from build123d import *

# Parameters (mm, degrees)
SKETCH1_W           = 130
SKETCH1_H           = 230
BOSS_EXTRUDE1_DEPTH = 2
EXTRUDE_THIN1_DEPTH = 0.5
SKETCH3_R           = 1.5
CUT_EXTRUDE1_DEPTH  = 133.113587492


with BuildPart() as part:
    # Sketch1 → Boss-Extrude1 (new body)
    with BuildSketch(Plane.XY):
        Rectangle(SKETCH1_W, SKETCH1_H)
    extrude(amount=BOSS_EXTRUDE1_DEPTH)

    # Sketch2 → Extrude-Thin1 (add)
    with BuildSketch(Plane.XY.offset(2)):
        with BuildLine():
            Line((58.95, 84.95), (63, 84.95))
            Line((63, 84.95), (63, -104.9))
            Line((63, -104.9), (58.95, -104.9))
            ThreePointArc((58.95, -104.9), (56.086217536, -106.086217536), (54.9, -108.95))
            Line((54.9, -108.95), (54.9, -113))
            Line((54.9, -113), (-54.9, -113))
            Line((-54.9, -113), (-54.9, -108.95))
            ThreePointArc((-54.9, -108.95), (-56.086217536, -106.086217536), (-58.95, -104.9))
            Line((-58.95, -104.9), (-63, -104.9))
            Line((-63, -104.9), (-63, 104.9))
            Line((-63, 104.9), (-58.95, 104.9))
            ThreePointArc((-58.95, 104.9), (-56.086217536, 106.086217536), (-54.9, 108.95))
            Line((-54.9, 108.95), (-54.9, 113))
            Line((-54.9, 113), (63, 113))
            Line((63, 113), (63, 93.05))
            Line((63, 93.05), (58.95, 93.05))
            ThreePointArc((58.95, 93.05), (54.9, 89), (58.95, 84.95))
        make_face()
        with BuildLine():
            Line((58.95, 83.95), (62, 83.95))
            Line((62, 83.95), (62, -103.9))
            Line((62, -103.9), (58.95, -103.9))
            ThreePointArc((58.95, -103.9), (55.379110755, -105.379110755), (53.9, -108.95))
            Line((53.9, -108.95), (53.9, -112))
            Line((53.9, -112), (-53.9, -112))
            Line((-53.9, -112), (-53.9, -108.95))
            ThreePointArc((-53.9, -108.95), (-55.379110755, -105.379110755), (-58.95, -103.9))
            Line((-58.95, -103.9), (-62, -103.9))
            Line((-62, -103.9), (-62, 103.9))
            Line((-62, 103.9), (-58.95, 103.9))
            ThreePointArc((-58.95, 103.9), (-55.379110755, 105.379110755), (-53.9, 108.95))
            Line((-53.9, 108.95), (-53.9, 112))
            Line((-53.9, 112), (62, 112))
            Line((62, 112), (62, 94.05))
            Line((62, 94.05), (58.95, 94.05))
            ThreePointArc((58.95, 94.05), (53.9, 89), (58.95, 83.95))
        make_face(mode=Mode.SUBTRACT)
    extrude(amount=EXTRUDE_THIN1_DEPTH)

    # Sketch3 → Cut-Extrude1 (cut, through all)
    with BuildSketch(Plane.XY.offset(2)):
        with Locations((59, -109)):
            Circle(SKETCH3_R)
        with Locations((-59, -109)):
            Circle(SKETCH3_R)
        with Locations((-59, 109)):
            Circle(SKETCH3_R)
        with Locations((59, 89)):
            Circle(SKETCH3_R)
    extrude(amount=-CUT_EXTRUDE1_DEPTH, mode=Mode.SUBTRACT)


solid = part.part
Can you work these out from the model? Positions are in its coordinate system, mm. A direction names the side the tool comes from. Round coordinates to 2 decimals unless told otherwise and drop trailing zeros. Write each loop counter-clockwise with the first axis right and the second up, starting at its lowest first coordinate (ties: lowest second). Pieces come first, ordered by that corner, then holes. Notation, with made-up numbers: (26.5, 83.5) -> (82.5, 83.5) arc R22 cw to (82.5, 94.5) -> close; hole circle Ø1 at (76, 11.5). An arc over 180 degrees is marked (long way). One line per question, with ' | ' between items. Start each with the question number.
1) I need wall thicknesses on line 1 (Y direction, x = -59, z = 1.45); line 2 (X direction, y = -109, z = 0.55); line 3 (Y direction, x = 59, z = 1.2). Which ranges of each line are inside material? Lowest first, please. Write a range as [from, to].
2) Suppose I cut it at A-A on y = 100. Write out the boundary of the cut face in (x, z).
3) I'm going to push flat-ended pins straight in: P1, Ø0.6, axis at y = -110, z = 2.5, coming from the -X side; P2, Ø0.6, axis at y = 35.5, z = 2.5, coming from the +X side. Where does each tip first touch, or does it pass through?
4) On a 3-axis mill with a long thin cutter (end or side, diameter ignored), from which of +Z, -Z, +X, -X, +Y, -Y can I reach the whole of each face in a straight line? I mean faces 1 (the cylindrical face through (-56.055, -106.118, 2.246)), 2 (the cylindrical face through (-55.42, 105.34, 2.25)), 3 (the cylindrical face through (54.9, 89.1, 2.2)), 4 (the cylindrical face through (-56.118, 106.055, 2.246)). Say none if no direction works.
5) Suppose I cut it at B-B on x = 10.5. Write out the boundary of the cut face in (y, z), then the cut area to 3 significant figures.
6) If we mould it in two halves opening along X, with no side actions, what happens to faces 5 (the cylindrical face through (55.42, -105.34, 2.25)), 6 (the cylindrical face through (-55.34, -105.42, 2.25)), 7 (the cylindrical face through (56.118, -106.055, 2.246)), 8 (the flat face through (-1, 2, 0))? For each: released by +X, released by -X, zero draft, split by the parting line, or undercut.
Return value:
1) line 1: y = [-115, -110.5], [-107.5, 107.5], [110.5, 115] | line 2: x = [-65, -60.5], [-57.5, 57.5], [60.5, 65] | line 3: y = [-115, -110.5], [-107.5, 87.5], [90.5, 115]
2) outline: (-65, 0) -> (65, 0) -> (65, 2) -> (63, 2) -> (63, 2.5) -> (62, 2.5) -> (62, 2) -> (-62, 2) -> (-62, 2.5) -> (-63, 2.5) -> (-63, 2) -> (-65, 2) -> close
3) P1: stops at x = -54.9 | P2: stops at x = 63
4) face 1: +Z, -X, -Y | face 2: +Z | face 3: +Z, +X | face 4: +Z, -X, +Y
5) outline: (-115, 0) -> (115, 0) -> (115, 2) -> (113, 2) -> (113, 2.5) -> (112, 2.5) -> (112, 2) -> (-112, 2) -> (-112, 2.5) -> (-113, 2.5) -> (-113, 2) -> (-115, 2) -> close | area: 461 mm2
6) face 5: undercut | face 6: undercut | face 7: released by +X | face 8: zero draft
